Geometry check sheet. Reference: the model listing, model coordinates, mm. Face numbers are marked on the shaded views. A direction names the side the tool comes from. Give positions to 0.01 mm unless a question says otherwise; leave off trailing zeros. Write each loop counter-clockwise with the first axis right and the second up, starting at its lowest first coordinate (ties: lowest second). Pieces come first, ordered by that corner, then holes. Notation, with made-up numbers: M 19.5,37.25 L 67.5,37.25 A17 cw 67.5,47.25 Z; hole C 12,79.25 d5. An arc over 180 degrees is marked long. One line per item, written item: value. Start each with the question number.
1. Cross-section at B-B on y = 70. Record the cut outline in (x, z).
2. Cross-section at C-C on x = 24.57. Record the cut outline in (y, z), then the cut area to 3 significant figures.
3. Cross-section at A-A on z = 54. Record the cut outline in (x, y).
4. Gauge pin test, flat ends, axial feed: pin 1 (6 mm diameter, centred on y = 127.5, z = 54, fed in from -X); pin 2 (0.9 mm diameter, centred on y = 3, z = 1, fed in from +X); pin 3 (6 mm diameter, centred on x = 22, y = 75.5, fed in from +Z). Record the tip position at first contact, or that the pin passes through.
5. Tool access check on the marked faces 1 and 2. Record the directions out of +Z, -Z, +X, -X, +Y, -Y that give a thin tool (end or side, any length) a straight path to the whole face; none if there is none.
6. Cross-section at D-D on y = 46.43. Record the cut outline in (x, z), then the cut area to 3 significant figures.
7. Scan lines: line 1 (Y direction, x = -33, z = 14); line 2 (Z direction, x = -33, y = 127); line 3 (X direction, y = 73.5, z = 57). Record each from-to range of solid material in increasing order.
from build123d import *

# Parameters (mm, degrees)
SKETCH1_W                    = 70
SKETCH1_H                    = 3
BASE_FLANGE1_DEPTH           = 140
EDGE_FLANGE1_STRIP_W         = 18
EDGE_FLANGE1_STRIP_H         = 3
EDGE_FLANGE1_STRIP_CUT_DEPTH = 140
EDGE_FLANGE1_DEPTH           = 140
SKETCH9_R                    = 19
SKETCH9_R_2                  = 3
CUT_EXTRUDE1_DEPTH           = 10
SKETCH10_R                   = 2.5
CUT_EXTRUDE2_DEPTH           = 10
SKETCH11_R                   = 2.5
CUT_EXTRUDE3_DEPTH           = 3
CUT_EXTRUDE4_DEPTH           = 10
FILLET1_R                    = 10
FILLET2_R                    = 10


# Sheet-metal steps are written as plain solids
with BuildPart() as part:
    # Sketch1 → Base-Flange1 (new body)
    with BuildSketch(Plane(origin=(0, 0, 0), x_dir=(1, 0, 0), z_dir=(0, 1, 0))):
        with Locations((0, -1.5)):
            Rectangle(SKETCH1_W, SKETCH1_H)
    extrude(amount=BASE_FLANGE1_DEPTH)

    # Edge-Flange1 strip (across the edge) → Edge-Flange1 strip cut (cut)
    with BuildSketch(Plane(origin=(-35, 140, 3), x_dir=(1, 0, 0), z_dir=(0, -1, 0))):
        with Locations((-3, -1.5)):
            Rectangle(EDGE_FLANGE1_STRIP_W, EDGE_FLANGE1_STRIP_H)
    extrude(amount=EDGE_FLANGE1_STRIP_CUT_DEPTH, mode=Mode.SUBTRACT)

    # Edge-Flange1 section (across the edge) → Edge-Flange1 (add)
    with BuildSketch(Plane(origin=(-35, 140, 3), x_dir=(1, 0, 0), z_dir=(0, -1, 0))):
        with BuildLine():
            Line((0, 3), (0, 61))
            Line((0, 61), (3, 61))
            Line((3, 61), (3, 3))
            ThreePointArc((3, 3), (3.878679656, 0.878679656), (6, 0))
            Line((6, 0), (6, -3))
            ThreePointArc((6, -3), (1.757359313, -1.242640687), (0, 3))
        make_face()
    extrude(amount=EDGE_FLANGE1_DEPTH)

    # Sketch9 → Cut-Extrude1 (cut)
    with BuildSketch(Plane.XY.offset(3)):
        with Locations((1, 70)):
            Circle(SKETCH9_R)
        with Locations((-22.57, 93.57)):
            Circle(SKETCH9_R_2)
        with Locations((24.57, 93.57)):
            Circle(SKETCH9_R_2)
        with Locations((24.57, 46.43)):
            Circle(SKETCH9_R_2)
        with Locations((-22.57, 46.43)):
            Circle(SKETCH9_R_2)
    extrude(amount=-CUT_EXTRUDE1_DEPTH, mode=Mode.SUBTRACT)

    # Sketch10 → Cut-Extrude2 (cut)
    with BuildSketch(Plane(origin=(-32, 0, 0), x_dir=(0, 0, -1), z_dir=(1, 0, 0))):
        with Locations((-54, 127.5)):
            Circle(SKETCH10_R)
        with Locations((-14, 127.5)):
            Circle(SKETCH10_R)
        with Locations((-14, 12.5)):
            Circle(SKETCH10_R)
        with Locations((-54, 12.5)):
            Circle(SKETCH10_R)
    extrude(amount=-CUT_EXTRUDE2_DEPTH, mode=Mode.SUBTRACT)

    # Sketch11 → Cut-Extrude3 (cut)
    with BuildSketch(Plane.XY.offset(3)):
        with Locations((0, 120)):
            Circle(SKETCH11_R)
        with Locations((0, 20)):
            Circle(SKETCH11_R)
    extrude(amount=-CUT_EXTRUDE3_DEPTH, mode=Mode.SUBTRACT)

    # Sketch12 → Cut-Extrude4 (cut)
    with BuildSketch(Plane(origin=(0, 0, 0), x_dir=(-1, 0, 0), z_dir=(0, 0, -1))):
        Polygon((-35, 95.130192279), (-35, 140), (29, 140), (29, 133.118302038), align=None)
        Polygon((29, 0), (29, 6.881697962), (-35, 44.869807721), (-35, 0), align=None)
    extrude(amount=-CUT_EXTRUDE4_DEPTH, mode=Mode.SUBTRACT)

    # Fillet1
    fillet1_edges = [part.edges().sort_by_distance(p)[0] for p in [
        (35, 44.869807721, 1.5),
    ]]
    fillet(fillet1_edges, radius=FILLET1_R)

    # Fillet2
    fillet2_edges = [part.edges().sort_by_distance(p)[0] for p in [
        (35, 95.130192279, 1.5),
    ]]
    fillet(fillet2_edges, radius=FILLET2_R)


solid = part.part
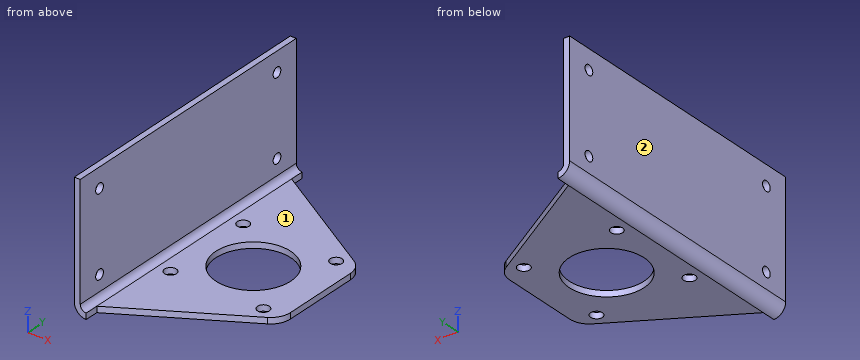
Report:
1. outline: M -35,6 A6 ccw -29,0 L -18,0 L -18,3 L -29,3 A3 cw -32,6 L -32,64 L -35,64 Z; M 20,0 L 35,0 L 35,3 L 20,3 Z
2. outline: M 38.68,0 L 43.43,0 L 43.43,3 L 38.68,3 Z; M 49.43,0 L 90.57,0 L 90.57,3 L 49.43,3 Z; M 96.57,0 L 101.32,0 L 101.32,3 L 96.57,3 Z
2. area: 152 mm^2
3. outline: M -35,0 L -32,0 L -32,10 L -35,10 Z; M -35,15 L -32,15 L -32,125 L -35,125 Z; M -35,130 L -32,130 L -32,140 L -35,140 Z
4. pin 1: stops at x = -35
4. pin 2: stops at x = -29
4. pin 3: stops at z = 3
5. face 1: +Z, +X, +Y, -Y
5. face 2: +Z, -Z, -X, +Y, -Y
6. outline: M -35,6 A6 ccw -29,0 L -25.57,0 L -25.57,3 L -29,3 A3 cw -32,6 L -32,64 L -35,64 Z; M -19.57,0 L 21.57,0 L 21.57,3 L -19.57,3 Z; M 27.57,0 L 34.11,0 L 34.11,3 L 27.57,3 Z
6. area: 349 mm^2
7. line 1: y = 0 to 10, 15 to 125, 130 to 140
7. line 2: z = 1.53 to 11.55, 16.45 to 51.55, 56.45 to 64
7. line 3: x = -35 to -32
